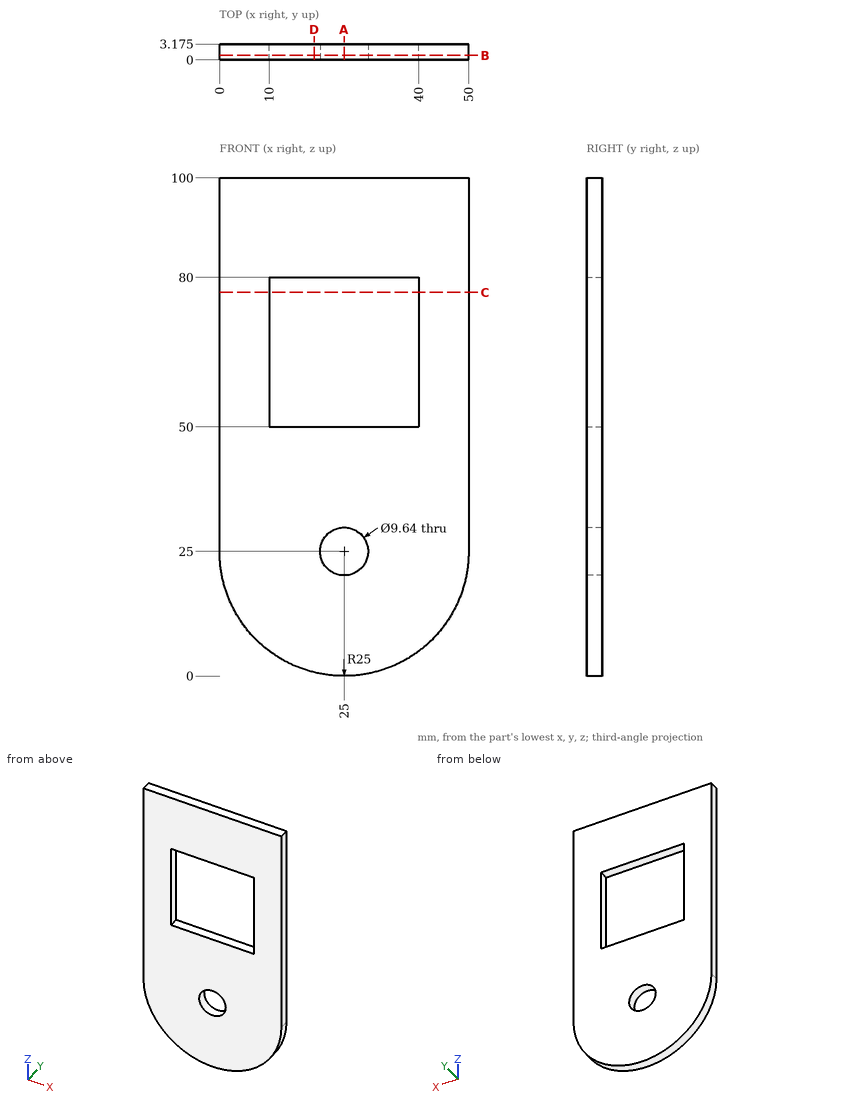
Design review of the part shown in the three views and the two pictorial views. Dimensions are in mm from the part's minimum x, y and z. Round coordinates to 2 decimals unless told otherwise and drop trailing zeros. Write each loop counter-clockwise with the first axis right and the second up, starting at its lowest first coordinate (ties: lowest second). Pieces come first, ordered by that corner, then holes. Notation, with made-up numbers: M -3.75,-16.75 L 4.25,-16.75 A20 ccw 4.25,-1.75 Z; hole C 22,-40 d5. An arc over 180 degrees is marked long. Use a Markdown table: item, result. Add a question column.
Q1. We need section D-D, the plane x = 19. State the section outline as (y, z) points (3 decimals), plus the area to 3 significant figures.
Q2. To check wall thickness, follow line 1 (X direction, y = 1.05, z = 25); line 2 (Z direction, x = 24, y = 2.6); line 3 (X direction, y = 1.6, z = 55). State the ranges of each line that lie inside material, in increasing order.
Q3. We need section A-A, the plane x = 25. State the section outline as (y, z) points (3 decimals).
Q4. Insertion check: pin 1 (1 mm diameter, centred on x = 5.5, z = 71, fed in from -Y); pin 2 (1 mm diameter, centred on x = 14.5, y = 1, fed in from -Z); pin 3 (1.5 mm diameter, centred on x = 29, y = 0.5, fed in from -Z). Each pin has a flat end and moves straight along its axis. Give the tip position at first contact, or say it passes through.
Q5. We need section B-B, the plane y = 0.9. State the section outline as (x, z) points.
Q6. We need section C-C, the plane z = 77. State the section outline as (x, y) points (3 decimals), plus the area to 3 significant figures.
Findings below:
| question | item | result |
|---|---|---|
| 1 | outline | M 0,0.731 L 3.175,0.731 L 3.175,50 L 0,50 Z; M 0,80 L 3.175,80 L 3.175,100 L 0,100 Z |
| 1 | area | 220 mm² |
| 2 | line 1 | x = 0 to 20.18, 29.82 to 50 |
| 2 | line 2 | z = 0.02 to 20.28, 29.72 to 50, 80 to 100 |
| 2 | line 3 | x = 0 to 10, 40 to 50 |
| 3 | outline | M 0,0 L 3.175,0 L 3.175,20.18 L 0,20.18 Z; M 0,29.82 L 3.175,29.82 L 3.175,50 L 0,50 Z; M 0,80 L 3.175,80 L 3.175,100 L 0,100 Z |
| 4 | pin 1 | stops at y = 0 |
| 4 | pin 2 | stops at z = 2.09 |
| 4 | pin 3 | stops at z = 0.21 |
| 5 | outline | M 0,25 A25 ccw 50,25 L 50,100 L 0,100 Z; hole M 10,50 L 40,50 L 40,80 L 10,80 Z; hole C 25,25 d9.64 |
| 6 | outline | M 0,0 L 10,0 L 10,3.175 L 0,3.175 Z; M 40,0 L 50,0 L 50,3.175 L 40,3.175 Z |
| 6 | area | 63.5 mm² |
